Work out the finished part from the listing and answer in its coordinate system (mm). Face numbers are marked on the shaded views. A direction names the side the tool comes from. Round coordinates to 2 decimals unless told otherwise and drop trailing zeros. Order: outer loops, then holes, each group sorted by start corner. A loop starts at its lowest first (then second) coordinate and runs counter-clockwise, first axis right, second up. Notation, with made-up numbers: (50, 82) - (56, 82) arc R30 ccw to (56, 104) - close; hole circle Ø10 at (78, -35). An arc over 180 degrees is marked (long way). Use one line per item in the form item = value. Start each with the question number.
Q1. The part is cut by section A-A on y = 4.5. Determine the outline of the cut face in (x, z), plus the area to 3 significant figures.
Q2. The part is cut by section C-C on y = 7. Determine the outline of the cut face in (x, z), plus the area to 3 significant figures.
Q3. The part is cut by section D-D on z = -1. Determine the outline of the cut face in (x, y), plus the area to 3 significant figures.
Q4. Which of the six approach directions +Z, -Z, +X, -X, +Y, -Y give full straight-line access (tool end or side, diameter ignored) to the marked faces 1, 2 and 3?
Q5. The part is cut by section B-B on x = 0. Determine the outline of the cut face in (y, z), plus the area to 3 significant figures.
Q6. Given P1, Ø1, axis at x = 1, z = 2, coming from the +Y side; P2, Ø4, axis at x = 0.5, y = 13.5, coming from the -Z side; P3, Ø1.5, axis at x = 1.5, y = 11, coming from the +Z side; P4, Ø3, axis at x = -0.5, z = 0.5, coming from the -Y side, each flat-ended and moving along its own axis, determine where each tip first touches the part or whether it passes through.
Q7. Find the intervals of material crossed by line 1 (Z direction, x = 0, y = 1.3); line 2 (Y direction, x = -0.5, z = 1); line 3 (Z direction, x = -1.5, y = 2.5), in increasing order. Write a range as [from, to].
Autodesk Inventor part; units mm, degrees
ref_plane "YZ Plane" through (0, 0, 0) normal (1, 0, 0) x (0, 1, 0)
ref_plane "XZ Plane" through (0, 0, 0) normal (0, 1, 0) x (-1, 0, 0)
ref_plane "XY Plane" through (0, 0, 0) normal (0, 0, 1) x (1, 0, 0)
sketch "Sketch1" plane through (0, 0, 0) normal (0, 1, 0) x (-1, 0, 0)
  line L0 (-3.4641, 0) -> (-1.7321, 3)
  line L1 (-1.7321, 3) -> (1.7321, 3)
  line L2 (1.7321, 3) -> (3.4641, 0)
  line L3 (3.4641, 0) -> (1.7321, -3)
  line L4 (1.7321, -3) -> (-1.7321, -3)
  line L5 (-1.7321, -3) -> (-3.4641, 0)
  point P0 (0, 0)
  point P1 (0, 0)
  dimension "d1" = 6
extrude "Extrusion1" add sketch "Sketch1" along normal blind 10
sketch "Sketch2" plane through (0, 0, 0) normal (0, -1, 0) x (1, 0, 0)
  circle A0 centre (0, 0) radius 1.75
  dimension "d4" = 3.5
sketch "Sketch3" plane through (0, 10, 0) normal (0, 1, 0) x (1, 0, 0)
  circle A0 centre (0, 0) radius 1.5
  dimension "d5" = 3
extrude "Extrusion2" add sketch "Sketch3" along normal blind 5.7
extrude "Extrusion3" cut sketch "Sketch2" against normal blind 6
thread "Thread1"
thread "Thread2"
properties part number "spacer1cm"
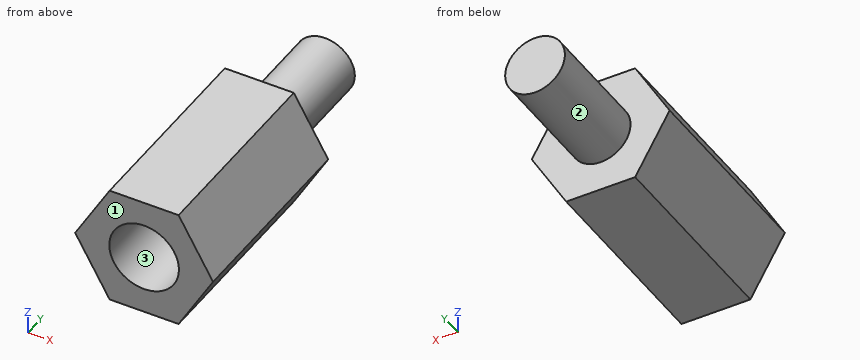
Found:
q1.outline = (-3.46, 0) - (-1.73, -3) - (1.73, -3) - (3.46, 0) - (1.73, 3) - (-1.73, 3) - close; hole circle Ø3.5 at (0, 0)
q1.area = 21.6 mm²
q2.outline = (-3.46, 0) - (-1.73, -3) - (1.73, -3) - (3.46, 0) - (1.73, 3) - (-1.73, 3) - close
q2.area = 31.2 mm²
q3.outline = (-2.89, 0) - (-1.44, 0) - (-1.44, 6) - (1.44, 6) - (1.44, 0) - (2.89, 0) - (2.89, 10) - (1.12, 10) - (1.12, 15.7) - (-1.12, 15.7) - (-1.12, 10) - (-2.89, 10) - close
q3.area = 53.2 mm²
q4.face_1 = +Z, -Z, +X, -X, -Y
q4.face_2 = +Y
q4.face_3 = -Y
q5.outline = (0, -3) - (10, -3) - (10, -1.5) - (15.7, -1.5) - (15.7, 1.5) - (10, 1.5) - (10, 3) - (0, 3) - (0, 1.75) - (6, 1.75) - (6, -1.75) - (0, -1.75) - close
q5.area = 56.1 mm²
q6.P1 = 10
q6.P2 = -1.5
q6.P3 = 1.3
q6.P4 = 0
q7.line_1 = [-3, -1.75], [1.75, 3]
q7.line_2 = [6, 15.7]
q7.line_3 = [-3, -0.9], [0.9, 3]
